Check sheet for the modelled part. Datum: model origin and axes. Units: mm. Coordinates: 2 decimals unless noted, no trailing zeros. Write each loop counter-clockwise with the first axis right and the second up, starting at its lowest first coordinate (ties: lowest second). Pieces come first, ordered by that corner, then holes. Notation, with made-up numbers: (8.5, -24) - (60.5, -24) arc R17 cw to (60.5, 8) - close; hole circle Ø1 at (81, 39). An arc over 180 degrees is marked (long way). Write each question's results on one line, items separated by ' | '.
from build123d import *

# Parameters (mm, degrees)
F0_R     = 5
F1_DEPTH = 127
F2_R     = 12.5
F2_R_2   = 5
F3_DEPTH = 10.16
F4_R     = 8.89


with BuildPart() as f1:
    # F0 (on Top) → F1 (new body)
    with BuildSketch(Plane.XY):
        Circle(F0_R)
    extrude(amount=F1_DEPTH)

    # F2 (on face) → F3 (join)
    with BuildSketch(Plane.XY.offset(127)):
        Circle(F2_R)
        Circle(F2_R_2, mode=Mode.SUBTRACT)
        Circle(F2_R_2)
    extrude(amount=F3_DEPTH)

    # F4
    f4_edges = [f1.edges().sort_by_distance(p)[0] for p in [
        (-12.5, 0, 137.16),
    ]]
    fillet(f4_edges, radius=F4_R)


solid = f1.part
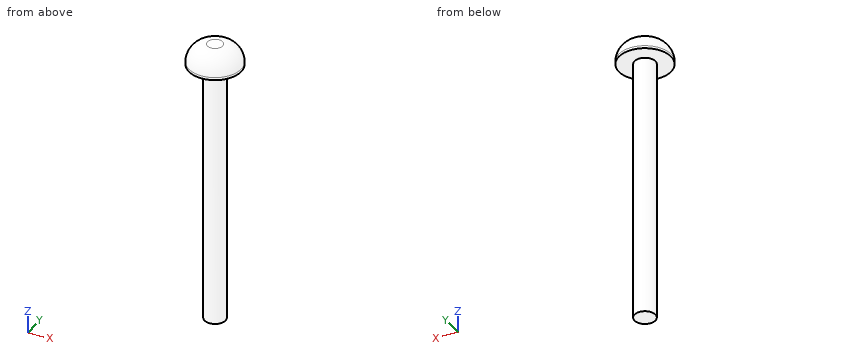
1. Go/stop test with flat-tipped pins: pin 1 (6 mm diameter, centred on x = -7, z = 87, fed in from +Y); pin 2 (1 mm diameter, centred on x = -2, z = 65.5, fed in from -Y); pin 3 (8 mm diameter, centred on x = -7.5, z = 32.5, fed in from -Y). Record where each tip stops, or that it passes through.
Values follow:
pin 1: stops at y = 3 | pin 2: stops at y = -4.77 | pin 3: stops at y = -3.57
2. Sectioned sample at A-A (z = 80). Record the cut outline in (x, y).
Values follow:
outline: circle Ø10 at (0, 0)
3. Material ranges on L1, parallel to X at y = -0.5, z = 98; L2, parallel to Z at x = -7, y = -5.75, recorded low to high. Write a range as [from, to].
Values follow:
L1: x = [-4.97, 4.97] | L2: z = [127, 135.29]
